Design review of the part built by this model. Coordinates are the model's own, in mm. A direction names the side the tool comes from. Coordinates: 2 decimals unless noted, no trailing zeros. Write each loop counter-clockwise with the first axis right and the second up, starting at its lowest first coordinate (ties: lowest second). Pieces come first, ordered by that corner, then holes.
Q1. Take a section at D-D (y = 1). Give the boundary of the cut face in (x, z).
Q2. Mouldability with a two-part tool opening along Z and no side actions: class faces 3 (the flat face through (-25.07, 4.965, 11.465)), 4 (the cylindrical face through (-19, 6, 0)), 5 (the flat face through (-24.93, 10.535, 0.196)) as pulls with the +Z half, pulls with the -Z half, needs draft (parallel to the pull), parting line crosses it, or undercut.
Q3. Take a section at A-A (x = -5). Give the boundary of the cut face in (y, z).
Q4. Machinability: for faces 1 (the cylindrical face through (19, 6, 0)), 2 (the flat face through (30, 6, 0)), which of the approach directions +Z, -Z, +X, -X, +Y, -Y give a long, thin tool a straight path to every point of the face, cutting with its end or side? Answer none if there is none.
Q5. Take a section at C-C (z = 0). Give the boundary of the cut face in (x, y).
Q6. Take a section at B-B (y = 11.25). Give the boundary of the cut face in (x, z), and give its area (3 significant figures).
Q7. For probe 1 along Z at (x, y) = (-12.5, 7.25); probe 2 along X at (y, z) = (10.25, -1.25); probe 3 along Z at (x, y) = (-16, 11.5), list the stretches that pass through material, from the lowest coordinate up.
```python
from build123d import *

# Parameters (mm, degrees)
BOSS_EXTRUDE1_DEPTH = 13
CUT_EXTRUDE1_DEPTH  = 44.0464865


with BuildPart() as part:
    # Sketch1 → Boss-Extrude1 (new body)
    with BuildSketch(Plane(origin=(0, 0, 0), x_dir=(1, 0, 0), z_dir=(0, 1, 0))):
        Polygon((-20, -14), (30, -14), (30, 14), (-20, 14), (-30, 9), (-30, -9), align=None)
        with BuildLine():
            Line((-12.5, 6.5), (12.5, 6.5))
            ThreePointArc((12.5, 6.5), (19, 0), (12.5, -6.5))
            Line((12.5, -6.5), (-12.5, -6.5))
            ThreePointArc((-12.5, -6.5), (-19, 0), (-12.5, 6.5))
        make_face(mode=Mode.SUBTRACT)
    extrude(amount=BOSS_EXTRUDE1_DEPTH)

    # Sketch2 → Cut-Extrude1 (cut, through all)
    with BuildSketch(Plane.XY.offset(14)):
        Polygon((-30, 13), (-20, 13), (-30, 8), align=None)
    extrude(amount=-CUT_EXTRUDE1_DEPTH, mode=Mode.SUBTRACT)


solid = part.part
```
Response:
1. outline: (-30, -9) - (-20, -14) - (30, -14) - (30, 14) - (-20, 14) - (-30, 9) - close; hole (-12.5, -6.5) - (12.5, -6.5) arc R6.5 ccw to (12.5, 6.5) - (-12.5, 6.5) arc R6.5 ccw to start
2. face 3: pulls with the +Z half
2. face 4: undercut
2. face 5: needs draft
3. outline: (0, -14) - (13, -14) - (13, -6.5) - (0, -6.5) - close; (0, 6.5) - (13, 6.5) - (13, 14) - (0, 14) - close
4. face 1: +Y, -Y
4. face 2: +Z, -Z, +X, +Y, -Y
5. outline: (-30, 0) - (-19, 0) - (-19, 13) - (-20, 13) - (-30, 8) - close; (19, 0) - (30, 0) - (30, 13) - (19, 13) - close
6. outline: (-23.5, -12.25) - (-20, -14) - (30, -14) - (30, 14) - (-20, 14) - (-23.5, 12.25) - close; hole (-12.5, -6.5) - (12.5, -6.5) arc R6.5 ccw to (12.5, 6.5) - (-12.5, 6.5) arc R6.5 ccw to start
6. area: 1,030 mm2
7. probe 1: z = -14 to -6.5, 6.5 to 14
7. probe 2: x = -25.5 to -18.88, 18.88 to 30
7. probe 3: z = -14 to -5.48, 5.48 to 14
